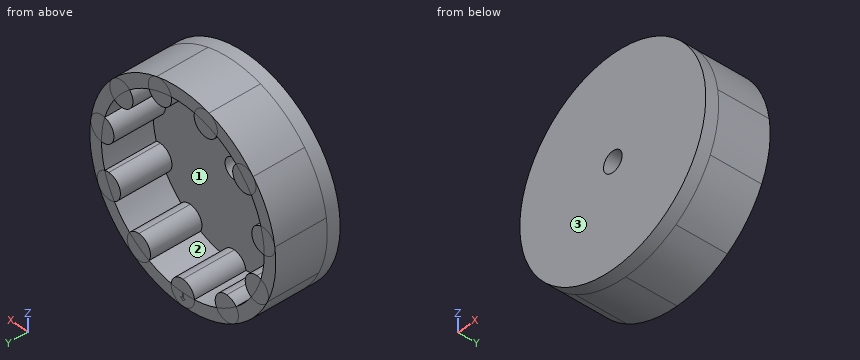
from build123d import *

# Parameters (mm, degrees)
SKETCH1_R              = 5
BOSS_EXTRUDE1_DEPTH    = 20
BOSS_EXTRUDE1_2_DEPTH  = 20
BOSS_EXTRUDE1_3_DEPTH  = 20
BOSS_EXTRUDE1_4_DEPTH  = 20
BOSS_EXTRUDE1_5_DEPTH  = 20
BOSS_EXTRUDE1_6_DEPTH  = 20
BOSS_EXTRUDE1_7_DEPTH  = 20
BOSS_EXTRUDE1_8_DEPTH  = 20
BOSS_EXTRUDE1_9_DEPTH  = 20
BOSS_EXTRUDE1_10_DEPTH = 20
BOSS_EXTRUDE1_11_DEPTH = 20
SKETCH2_R              = 35
SKETCH2_R_2            = 4
BOSS_EXTRUDE2_DEPTH    = 5
SKETCH3_W              = 0.25
SKETCH3_H              = 1.939339828
CUT_EXTRUDE1_DEPTH     = 0.1
BOSS_EXTRUDE4_START    = -5
SKETCH4_R              = 40
SKETCH4_R_2            = 35
BOSS_EXTRUDE4_DEPTH    = 5
BOSS_EXTRUDE5_START    = 20
SKETCH5_R              = 40
SKETCH5_R_2            = 35
BOSS_EXTRUDE5_DEPTH    = 20


with BuildPart() as part:
    # Sketch1 → Boss-Extrude1 (new body)
    with BuildSketch(Plane(origin=(0, 0, 0), x_dir=(1, 0, 0), z_dir=(0, 1, 0))):
        with Locations(Location((0, 35, 0), (0, 0, 270))):
            Circle(SKETCH1_R)
    extrude(amount=BOSS_EXTRUDE1_DEPTH)



with BuildPart() as body_2:
    # Sketch1 → Boss-Extrude1 2 (new body)
    with BuildSketch(Plane(origin=(0, 0, 0), x_dir=(1, 0, 0), z_dir=(0, 1, 0))):
        with Locations(Location((18.922428611, 29.443873649, 0), (0, 0, 270))):
            Circle(SKETCH1_R)
    extrude(amount=BOSS_EXTRUDE1_2_DEPTH)


with BuildPart() as body_3:
    # Sketch1 → Boss-Extrude1 3 (new body)
    with BuildSketch(Plane(origin=(0, 0, 0), x_dir=(1, 0, 0), z_dir=(0, 1, 0))):
        with Locations(Location((31.837119837, 14.539525455, 0), (0, 0, 270))):
            Circle(SKETCH1_R)
    extrude(amount=BOSS_EXTRUDE1_3_DEPTH)


with BuildPart() as body_4:
    # Sketch1 → Boss-Extrude1 4 (new body)
    with BuildSketch(Plane(origin=(0, 0, 0), x_dir=(1, 0, 0), z_dir=(0, 1, 0))):
        with Locations(Location((34.643750466, -4.98101934, 0), (0, 0, 270))):
            Circle(SKETCH1_R)
    extrude(amount=BOSS_EXTRUDE1_4_DEPTH)


with BuildPart() as body_5:
    # Sketch1 → Boss-Extrude1 5 (new body)
    with BuildSketch(Plane(origin=(0, 0, 0), x_dir=(1, 0, 0), z_dir=(0, 1, 0))):
        with Locations(Location((26.451235102, -22.920125688, 0), (0, 0, 270))):
            Circle(SKETCH1_R)
    extrude(amount=BOSS_EXTRUDE1_5_DEPTH)


with BuildPart() as body_6:
    # Sketch1 → Boss-Extrude1 6 (new body)
    with BuildSketch(Plane(origin=(0, 0, 0), x_dir=(1, 0, 0), z_dir=(0, 1, 0))):
        with Locations(Location((9.860639489, -33.582254077, 0), (0, 0, 270))):
            Circle(SKETCH1_R)
    extrude(amount=BOSS_EXTRUDE1_6_DEPTH)


with BuildPart() as body_7:
    # Sketch1 → Boss-Extrude1 7 (new body)
    with BuildSketch(Plane(origin=(0, 0, 0), x_dir=(1, 0, 0), z_dir=(0, 1, 0))):
        with Locations(Location((-9.860639489, -33.582254077, 0), (0, 0, 270))):
            Circle(SKETCH1_R)
    extrude(amount=BOSS_EXTRUDE1_7_DEPTH)


with BuildPart() as body_8:
    # Sketch1 → Boss-Extrude1 8 (new body)
    with BuildSketch(Plane(origin=(0, 0, 0), x_dir=(1, 0, 0), z_dir=(0, 1, 0))):
        with Locations(Location((-26.451235102, -22.920125688, 0), (0, 0, 270))):
            Circle(SKETCH1_R)
    extrude(amount=BOSS_EXTRUDE1_8_DEPTH)


with BuildPart() as body_9:
    # Sketch1 → Boss-Extrude1 9 (new body)
    with BuildSketch(Plane(origin=(0, 0, 0), x_dir=(1, 0, 0), z_dir=(0, 1, 0))):
        with Locations(Location((-34.643750466, -4.98101934, 0), (0, 0, 270))):
            Circle(SKETCH1_R)
    extrude(amount=BOSS_EXTRUDE1_9_DEPTH)


with BuildPart() as body_10:
    # Sketch1 → Boss-Extrude1 10 (new body)
    with BuildSketch(Plane(origin=(0, 0, 0), x_dir=(1, 0, 0), z_dir=(0, 1, 0))):
        with Locations(Location((-31.837119837, 14.539525455, 0), (0, 0, 270))):
            Circle(SKETCH1_R)
    extrude(amount=BOSS_EXTRUDE1_10_DEPTH)


with BuildPart() as body_11:
    # Sketch1 → Boss-Extrude1 11 (new body)
    with BuildSketch(Plane(origin=(0, 0, 0), x_dir=(1, 0, 0), z_dir=(0, 1, 0))):
        with Locations(Location((-18.922428611, 29.443873649, 0), (0, 0, 270))):
            Circle(SKETCH1_R)
    extrude(amount=BOSS_EXTRUDE1_11_DEPTH)


with BuildPart() as part_1:
    add(part.part)

    add(body_2.part)  # Boss-Extrude2 merges body 2

    add(body_3.part)  # Boss-Extrude2 merges body 3

    add(body_4.part)  # Boss-Extrude2 merges body 4

    add(body_5.part)  # Boss-Extrude2 merges body 5

    add(body_6.part)  # Boss-Extrude2 merges body 6

    add(body_7.part)  # Boss-Extrude2 merges body 7

    add(body_8.part)  # Boss-Extrude2 merges body 8

    add(body_9.part)  # Boss-Extrude2 merges body 9

    add(body_10.part)  # Boss-Extrude2 merges body 10

    add(body_11.part)  # Boss-Extrude2 merges body 11
    # Sketch2 → Boss-Extrude2 (add)
    with BuildSketch(Plane(origin=(0, 0, 0), x_dir=(1, 0, 0), z_dir=(0, 1, 0))):
        with Locations(Location((0, 0, 0), (0, 0, 270))):
            Circle(SKETCH2_R)
        with Locations(Location((0, 0, 0), (0, 0, 270))):
            Circle(SKETCH2_R_2, mode=Mode.SUBTRACT)
    extrude(amount=-BOSS_EXTRUDE2_DEPTH)

    # Sketch3 → Cut-Extrude1 (cut)
    with BuildSketch(Plane(origin=(0, 20, 0), x_dir=(1, 0, 0), z_dir=(0, 1, 0))):
        Polygon((-1.060660172, 36.939339828), (-0.25, 36.939339828), (-0.25, 37.75), align=None)
        Polygon((-0.25, 36.939339828), (0, 36.939339828), (0, 38), (-0.25, 37.75), align=None)
        Polygon((0, 38), (0, 36.939339828), (0.25, 36.939339828), (0.25, 37.75), align=None)
        Polygon((0.25, 37.75), (0.25, 36.939339828), (1.060660172, 36.939339828), align=None)
        with Locations((0.125, 35.969669914)):
            Rectangle(SKETCH3_W, SKETCH3_H)
        with Locations((-0.125, 35.969669914)):
            Rectangle(SKETCH3_W, SKETCH3_H)
    extrude(amount=-CUT_EXTRUDE1_DEPTH, mode=Mode.SUBTRACT)

    # Sketch4 → Boss-Extrude4 (add)
    with BuildSketch(Plane.XZ.offset(5).offset(BOSS_EXTRUDE4_START)):
        with Locations(Location((0, 0, 0), (0, 0, 270))):
            Circle(SKETCH4_R)
        Circle(SKETCH4_R_2, mode=Mode.SUBTRACT)
    extrude(amount=BOSS_EXTRUDE4_DEPTH)

    # Sketch5 → Boss-Extrude5 (add)
    with BuildSketch(Plane(origin=(0, 0, 0), x_dir=(1, 0, 0), z_dir=(0, 1, 0)).offset(BOSS_EXTRUDE5_START)):
        with Locations(Location((0, 0, 0), (0, 0, 90))):
            Circle(SKETCH5_R)
        Circle(SKETCH5_R_2, mode=Mode.SUBTRACT)
    extrude(amount=-BOSS_EXTRUDE5_DEPTH)


solid = part_1.part
The model under review builds one solid part; all positions refer to its coordinate system, in mm. Face numbers are marked on the shaded views. Round coordinates to 2 decimals unless told otherwise and drop trailing zeros. Loops run counter-clockwise (first coordinate to the right, second up) from the corner with the lowest first, then second, coordinate; pieces in that order, holes last. Notation, with made-up numbers: (-27, 63.5) -> (0, 63.5) arc R20 ccw to (0, 67.5) -> close; hole circle Ø1 at (48.5, 34). An arc over 180 degrees is marked (long way). Return JSON: item names as keys, results as strings.
(1) Add section C-C on z = 15.5. Write out the cut boundary in (x, y).
Solved:
{"outline": "(-36.87, -5) -> (36.87, -5) -> (36.87, 20) -> (31.38, 20) -> (31.38, 0) -> (-31.38, 0) -> (-31.38, 20) -> (-36.87, 20) -> close"}
(2) The part is to be moulded in two halves that separate along X. For the marked faces 1, 2 and 3, say which applies: released by +X, released by -X, zero draft, split by the parting line, or undercut.
Solved:
{"face 1": "undercut", "face 2": "undercut", "face 3": "zero draft"}
(3) Add section B-B on x = -2. Write out the cut boundary in (y, z).
Solved:
{"outline": "(-5, -39.95) -> (20, -39.95) -> (20, -30.42) -> (0, -30.42) -> (0, -3.46) -> (-5, -3.46) -> close; (-5, 3.46) -> (0, 3.46) -> (0, 34.94) -> (20, 34.94) -> (20, 39.95) -> (-5, 39.95) -> close"}
(4) For pin 1 (12 mm diameter, centred on y = 8, z = 19, fed in from +X); pin 2 (1 mm diameter, centred on y = 3, z = -30.5, fed in from +X); pin 3 (5 mm diameter, centred on y = 11, z = 14, fed in from -X), all flat-tipped, find the tip position at first contact; note any pin that passes through.
Solved:
{"pin 1": "x = 37.83", "pin 2": "x = 26.46", "pin 3": "x = -38.31"}
(5) Add section A-A on y = 3.5. Write out the cut boundary in (x, z), plus the area to 3 significant figures.
Solved:
{"outline": "circle Ø80 at (0, 0); hole (-35, -0.01) arc R35 ccw to (-33.58, -9.85) arc R5 cw to (-29.44, -18.93) arc R35 ccw to (-22.92, -26.45) arc R5 cw to (-14.53, -31.84) arc R35 ccw to (-4.99, -34.64) arc R5 cw to (4.99, -34.64) arc R35 ccw to (14.53, -31.84) arc R5 cw to (22.92, -26.45) arc R35 ccw to (29.44, -18.93) arc R5 cw to (33.58, -9.85) arc R35 ccw to (35, -0.01) arc R5 cw to (33.58, 9.87) arc R35 ccw to (29.45, 18.92) arc R5 cw to (22.92, 26.46) arc R35 ccw to (14.55, 31.83) arc R5 cw to (4.97, 34.64) arc R35 ccw to (-4.97, 34.64) arc R5 cw to (-14.55, 31.83) arc R35 ccw to (-22.92, 26.46) arc R5 cw to (-29.45, 18.92) arc R35 ccw to (-33.58, 9.87) arc R5 cw to start", "area": "1,600 mm2"}
(6) For line 1 (X direction, y = -3.85, z = 0); line 2 (Z direction, x = 15, y = 18.5); line 3 (Z direction, x = -25, y = 12), list the stretches that pass through material, from the lowest coordinate up.
Solved:
{"line 1": "-40 to -4, 4 to 40", "line 2": "-37.08 to -26.34, 31.62 to 37.08", "line 3": "-31.22 to -24.49, 18.14 to 31.22"}
(7) Add section D-D on z = 24. Write out the cut boundary in (x, y), plus the area to 3 significant figures.
Solved:
{"outline": "(-32, -5) -> (32, -5) -> (32, 20) -> (21.57, 20) -> (21.57, 0) -> (-21.57, 0) -> (-21.57, 20) -> (-32, 20) -> close", "area": "737 mm2"}
